The listing builds one solid part. Answer for the finished solid, in the listing's coordinates (mm). Face numbers are marked on the shaded views. A direction names the side the tool comes from. Coordinates: 2 decimals unless noted, no trailing zeros. Order: outer loops, then holes, each group sorted by start corner. A loop starts at its lowest first (then second) coordinate and runs counter-clockwise, first axis right, second up. Notation, with made-up numbers: (83, 48) - (115, 48) arc R22 cw to (115, 59) - close; hole circle Ø1 at (-23, 18.5). An arc over 180 degrees is marked (long way). Use a Markdown table: item, result. Add a question column.
Item 1: The part is cut by section A-A, the plane x = -30.5. Give the vertices of the cut face in (y, z).
Item 2: Flat-ended cylindrical pins translate along their axes: P1, Ø4, axis at x = -32.5, y = 35, coming from the -Z side; P2, Ø5, axis at x = -29.5, z = 0, coming from the -Y side; P3, Ø3, axis at x = -27, y = 15, coming from the +Z side; P4, Ø4, axis at y = 20, z = -3.5, coming from the -X side. Find the tip coordinate at first contact, or state that the pin passes through.
Item 3: The part is cut by section D-D, the plane y = 30. Give the vertices of the cut face in (x, z).
Item 4: The part is cut by section B-B, the plane z = -2. Give the vertices of the cut face in (x, y).
Item 5: The part is cut by section C-C, the plane z = -7.5. Give the vertices of the cut face in (x, y).
Item 6: For the marked faces 1 and 2, determine the directions among +Z, -Z, +X, -X, +Y, -Y from which every point of the face is accessible in a straight line to the end or side of a thin tool.
Item 7: Find the intervals of material crossed by line 1 along Y through (x, z) = (-29.75, -6.75); line 2 along X through (y, z) = (23.5, -3.75); line 3 along Z through (x, y) = (-26.5, 38.5), in increasing order.
from build123d import *

# Parameters (mm, degrees)
SKETCH_2_W      = 10
SKETCH_2_H      = 10
EXTRUDE_2_DEPTH = 10
SKETCH_3_R      = 3
EXTRUDE_3_DEPTH = 40


with BuildPart() as part:
    # 草图2 → 凸台-拉伸2 (new body)
    with BuildSketch(Plane(origin=(0, 0, 0), x_dir=(1, 0, 0), z_dir=(0, 1, 0))):
        with Locations((-28.987967914, 3.735294118)):
            Rectangle(SKETCH_2_W, SKETCH_2_H)
    extrude(amount=EXTRUDE_2_DEPTH)

    # 草图3 → 凸台-拉伸3 (add)
    with BuildSketch(Plane(origin=(0, 10, 0), x_dir=(1, 0, 0), z_dir=(0, 1, 0))):
        with Locations(Location((-28.987967914, 3.735294118, 0), (0, 0, 270))):
            Circle(SKETCH_3_R)
    extrude(amount=EXTRUDE_3_DEPTH)


solid = part.part
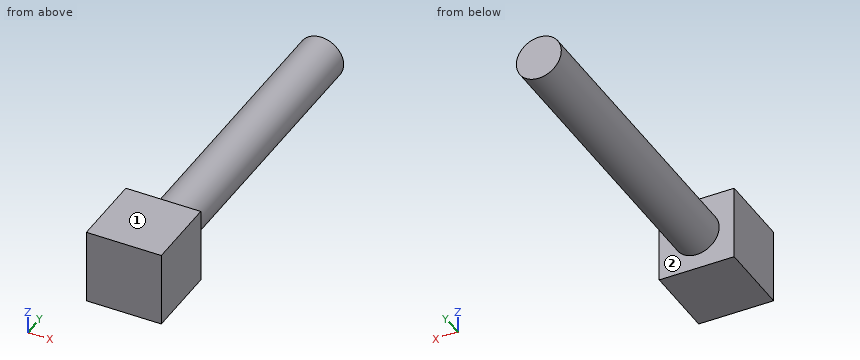
Solution:
| question | item | result |
|---|---|---|
| 1 | outline | (0, -8.74) - (10, -8.74) - (10, -6.33) - (50, -6.33) - (50, -1.14) - (10, -1.14) - (10, 1.26) - (0, 1.26) - close |
| 2 | P1 | stops at z = -6.33 |
| 2 | P2 | stops at y = 0 |
| 2 | P3 | stops at z = -0.78 |
| 2 | P4 | stops at x = -31.99 |
| 3 | outline | circle Ø6 at (-28.99, -3.74) |
| 4 | outline | (-33.99, 0) - (-23.99, 0) - (-23.99, 10) - (-26.54, 10) - (-26.54, 50) - (-31.44, 50) - (-31.44, 10) - (-33.99, 10) - close |
| 5 | outline | (-33.99, 0) - (-23.99, 0) - (-23.99, 10) - (-33.99, 10) - close |
| 6 | face 1 | +Z, +X, -X, +Y, -Y |
| 6 | face 2 | +Y |
| 7 | line 1 | y = 0 to 10 |
| 7 | line 2 | x = -31.99 to -25.99 |
| 7 | line 3 | z = -5.41 to -2.06 |
